Drawing for the job (mm, zero at the part's lowest x, y, z). Round coordinates to 2 decimals unless told otherwise and drop trailing zeros. Write each loop counter-clockwise with the first axis right and the second up, starting at its lowest first coordinate (ties: lowest second). Pieces come first, ordered by that corner, then holes. Notation, with made-up numbers: (70, 23.25) - (98, 23.25) arc R37 cw to (98, 62.25) - close; hole circle Ø4 at (68, -9.5). An arc over 180 degrees is marked (long way). Answer in a Markdown table with one row per item.
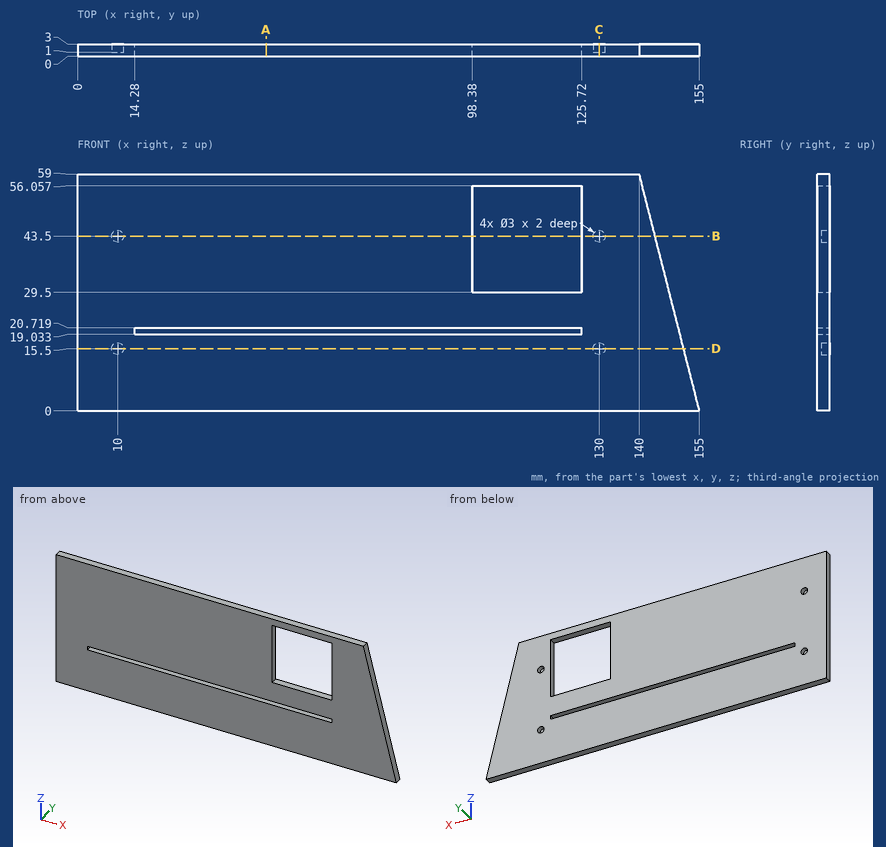
Q1. Drill centre lines: line 1 (Z direction, x = 130, y = 2.5); line 2 (Z direction, x = 106, y = 2.6); line 3 (Z direction, x = 60.5, y = 2.45). Where is each one in solid material? Low to high.
Computed:
| item | result |
|---|---|
| line 1 | z = 0 to 14, 17 to 42, 45 to 59 |
| line 2 | z = 0 to 19.03, 20.72 to 29.5, 56.06 to 59 |
| line 3 | z = 0 to 19.03, 20.72 to 59 |
Q2. Flat gauge pin, fed straight in: pin 1 (0.9 mm diameter, centred on x = 10, z = 16, fed in from +Y). Where does the tip first touch, or does it go through?
Computed:
| item | result |
|---|---|
| pin 1 | stops at y = 1 |
Q3. Saw through at A-A on x = 47. List the corners of the cut face in (y, z), then the cut area to 3 significant figures.
Computed:
| item | result |
|---|---|
| outline | (0, 0) - (3, 0) - (3, 19.03) - (0, 19.03) - close; (0, 20.72) - (3, 20.72) - (3, 59) - (0, 59) - close |
| area | 172 mm2 |
Q4. Saw through at C-C on x = 130. List the corners of the cut face in (y, z).
Computed:
| item | result |
|---|---|
| outline | (0, 0) - (3, 0) - (3, 14) - (1, 14) - (1, 17) - (3, 17) - (3, 42) - (1, 42) - (1, 45) - (3, 45) - (3, 59) - (0, 59) - close |
Q5. Saw through at B-B on z = 43.5. List the corners of the cut face in (x, y), then the cut area to 3 significant figures.
Computed:
| item | result |
|---|---|
| outline | (0, 0) - (98.38, 0) - (98.38, 3) - (11.5, 3) - (11.5, 1) - (8.5, 1) - (8.5, 3) - (0, 3) - close; (125.72, 0) - (143.94, 0) - (143.94, 3) - (131.5, 3) - (131.5, 1) - (128.5, 1) - (128.5, 3) - (125.72, 3) - close |
| area | 338 mm2 |
Q6. Saw through at D-D on z = 15.5. List the corners of the cut face in (x, y).
Computed:
| item | result |
|---|---|
| outline | (0, 0) - (151.06, 0) - (151.06, 3) - (131.5, 3) - (131.5, 1) - (128.5, 1) - (128.5, 3) - (11.5, 3) - (11.5, 1) - (8.5, 1) - (8.5, 3) - (0, 3) - close |
